Part model, mm, in its own coordinate system. Give positions to 0.01 mm unless a question says otherwise; leave off trailing zeros. Write each loop counter-clockwise with the first axis right and the second up, starting at its lowest first coordinate (ties: lowest second). Pieces come first, ordered by that corner, then holes.
```python
from build123d import *

# Parameters (mm, degrees)
SKETCH1_R                                    = 1.5
SKETCH1_R_2                                  = 3
BOSS_EXTRUDE1_DEPTH                          = 1.5
CSK_FOR_M1_6_COUNTERSUNK_FLAT_HEAD_S_2_COUNT = 2
CSK_FOR_M1_6_COUNTERSUNK_FLAT_HEAD_S_2_PITCH = 15.5
CSK_FOR_M1_6_COUNTERSUNK_FLAT_HEAD_S_3_COUNT = 2
CSK_FOR_M1_6_COUNTERSUNK_FLAT_HEAD_S_3_PITCH = 58.25
CSK_FOR_M1_6_COUNTERSUNK_FLAT_HEAD_S_4_COUNT = 2
CSK_FOR_M1_6_COUNTERSUNK_FLAT_HEAD_S_4_PITCH = 50.75


with BuildPart() as part:
    # Sketch1 → Boss-Extrude1 (new body)
    with BuildSketch(Plane.XY):
        with BuildLine():
            Line((15.5, 5.5), (-55, 5.5))
            ThreePointArc((-55, 5.5), (-60.5, 0), (-55, -5.5))
            Line((-55, -5.5), (15.5, -5.5))
            ThreePointArc((15.5, -5.5), (21, 0), (15.5, 5.5))
        make_face()
        with Locations((-55, 0)):
            Circle(SKETCH1_R, mode=Mode.SUBTRACT)
        Circle(SKETCH1_R_2, mode=Mode.SUBTRACT)
        with Locations((15.5, 0)):
            Circle(SKETCH1_R_2, mode=Mode.SUBTRACT)
    extrude(amount=BOSS_EXTRUDE1_DEPTH)

    # Sketch2 → CSK for M1.6 Countersunk Flat Head Screw1 (revolve, cut)
    with BuildSketch(Plane(origin=(7.75, 2.5, 1.5), x_dir=(0, -1, 0), z_dir=(1, 0, 0))):
        Polygon((0, 0), (0, 1.5), (0.9, 1.5), (0.9, 0.9), (1.8, 0), align=None)
    csk_for_m1_6_countersunk_flat_head_screw = revolve(axis=Axis((7.75, 2.5, 7.85), (0, 0, -1)), mode=Mode.SUBTRACT)

    # CSK for M1.6 Countersunk Flat Head S 2: CSK for M1.6 Countersunk Flat Head Screw1 ×2
    with Locations(*[(-i * CSK_FOR_M1_6_COUNTERSUNK_FLAT_HEAD_S_2_PITCH, 0, 0) for i in range(1, CSK_FOR_M1_6_COUNTERSUNK_FLAT_HEAD_S_2_COUNT)]):
        add(csk_for_m1_6_countersunk_flat_head_screw, mode=Mode.SUBTRACT)

    # CSK for M1.6 Countersunk Flat Head S 3: CSK for M1.6 Countersunk Flat Head Screw1 ×2
    with Locations(*[(-i * CSK_FOR_M1_6_COUNTERSUNK_FLAT_HEAD_S_3_PITCH, 0, 0) for i in range(1, CSK_FOR_M1_6_COUNTERSUNK_FLAT_HEAD_S_3_COUNT)]):
        add(csk_for_m1_6_countersunk_flat_head_screw, mode=Mode.SUBTRACT)

    # CSK for M1.6 Countersunk Flat Head S 4: CSK for M1.6 Countersunk Flat Head Screw1 ×2
    with Locations(*[(-i * CSK_FOR_M1_6_COUNTERSUNK_FLAT_HEAD_S_4_PITCH, 0, 0) for i in range(1, CSK_FOR_M1_6_COUNTERSUNK_FLAT_HEAD_S_4_COUNT)]):
        add(csk_for_m1_6_countersunk_flat_head_screw, mode=Mode.SUBTRACT)

    # Mirror1: CSK for M1.6 Countersunk Flat Head Screw1 across plane
    add(csk_for_m1_6_countersunk_flat_head_screw.mirror(Plane.ZX), mode=Mode.SUBTRACT)

    # Mirror1 copy 1 sketch → Mirror1 copy 1 (revolve, cut)
    with BuildSketch(Plane(origin=(-7.75, -2.5, 1.5), x_dir=(0, 1, 0), z_dir=(1, 0, 0))):
        Polygon((0, 0), (0, -1.5), (0.9, -1.5), (0.9, -0.9), (1.8, 0), align=None)
    revolve(axis=Axis((-7.75, -2.5, 7.85), (0, 0, 1)), mode=Mode.SUBTRACT)

    # Mirror1 copy 2 sketch → Mirror1 copy 2 (revolve, cut)
    with BuildSketch(Plane(origin=(-50.5, -2.5, 1.5), x_dir=(0, 1, 0), z_dir=(1, 0, 0))):
        Polygon((0, 0), (0, -1.5), (0.9, -1.5), (0.9, -0.9), (1.8, 0), align=None)
    revolve(axis=Axis((-50.5, -2.5, 7.85), (0, 0, 1)), mode=Mode.SUBTRACT)

    # Mirror1 copy 3 sketch → Mirror1 copy 3 (revolve, cut)
    with BuildSketch(Plane(origin=(-43, -2.5, 1.5), x_dir=(0, 1, 0), z_dir=(1, 0, 0))):
        Polygon((0, 0), (0, -1.5), (0.9, -1.5), (0.9, -0.9), (1.8, 0), align=None)
    revolve(axis=Axis((-43, -2.5, 7.85), (0, 0, 1)), mode=Mode.SUBTRACT)


solid = part.part
```
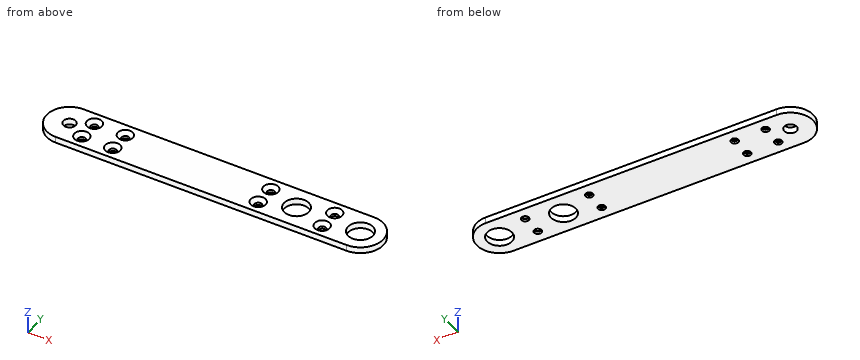
1) Saw through at D-D, the plane y = 0. Write the cut outline in (x, z), then the cut area to 4 significant figures.
Answers follow:
outline: (-60.5, 0) - (-56.5, 0) - (-56.5, 1.5) - (-60.5, 1.5) - close; (-53.5, 0) - (-3, 0) - (-3, 1.5) - (-53.5, 1.5) - close; (3, 0) - (12.5, 0) - (12.5, 1.5) - (3, 1.5) - close; (18.5, 0) - (21, 0) - (21, 1.5) - (18.5, 1.5) - close
area: 99.75 mm2
2) Pin check, flat tips, straight feed: pin 1 Ø1.1 at (x, y) = (-50.5, 2.5) entering from -Z; pin 2 Ø2.5 at (x, y) = (-7.75, -2.5) entering from +Z. Stop position of each tip, or through.
Answers follow:
pin 1: passes through
pin 2: stops at z = 0.95
3) Wall check: L1, parallel to Y at x = 7.75, z = 0.2; L2, parallel to X at y = -3.25, z = 1.25; L3, parallel to X at y = 3.25, z = 0.6. Give the ranges that are in metal, low to high.
Answers follow:
L1: y = -5.5 to -3.4, -1.6 to 1.6, 3.4 to 5.5
L2: x = -59.44 to -51.86, -49.14 to -44.36, -41.64 to -9.11, -6.39 to 6.39, 9.11 to 19.94
L3: x = -59.44 to -51, -50 to -43.5, -42.5 to -8.25, -7.25 to 7.25, 8.25 to 19.94
4) Saw through at A-A, the plane x = -43. Write the cut outline in (y, z).
Answers follow:
outline: (-5.5, 0) - (-3.4, 0) - (-3.4, 0.6) - (-4.3, 1.5) - (-5.5, 1.5) - close; (-1.6, 0) - (1.6, 0) - (1.6, 0.6) - (0.7, 1.5) - (-0.7, 1.5) - (-1.6, 0.6) - close; (3.4, 0) - (5.5, 0) - (5.5, 1.5) - (4.3, 1.5) - (3.4, 0.6) - close
5) Saw through at B-B, the plane z = 0.35. Count the separate pieces of the cut face and the enclosed holes in it, then the cut area to 3 significant figures.
Answers follow:
separate pieces: 1
enclosed holes: 11
area: 787 mm2
6) Saw through at C-C, the plane x = 0. Write the cut outline in (y, z), then the cut area to 3 significant figures.
Answers follow:
outline: (-5.5, 0) - (-3, 0) - (-3, 1.5) - (-5.5, 1.5) - close; (3, 0) - (5.5, 0) - (5.5, 1.5) - (3, 1.5) - close
area: 7.50 mm2
